The listing builds one solid part. Answer for the finished solid, in the listing's coordinates (mm). Face numbers are marked on the shaded views. Coordinates: 2 decimals unless noted, no trailing zeros. Loops run counter-clockwise (first coordinate to the right, second up) from the corner with the lowest first, then second, coordinate; pieces in that order, holes last. Notation, with made-up numbers: (52.5, -11.5) - (102.5, -11.5) arc R10 ccw to (102.5, -1.5) - close; hole circle Ø9 at (-6, -29). An arc over 180 degrees is marked (long way). One line per question, with ' | ' between items.
from build123d import *

# Parameters (mm, degrees)
SKETCH1_R           = 1.5
BOSS_EXTRUDE1_DEPTH = 7


with BuildPart() as part:
    # Sketch1 → Boss-Extrude1 (new body)
    with BuildSketch(Plane(origin=(0, 0, 0), x_dir=(1, 0, 0), z_dir=(0, 1, 0))):
        Polygon((2.886751346, 0), (1.443375673, 2.5), (-1.443375673, 2.5), (-2.886751346, 0), (-1.443375673, -2.5), (1.443375673, -2.5), align=None)
        Circle(SKETCH1_R, mode=Mode.SUBTRACT)
    extrude(amount=BOSS_EXTRUDE1_DEPTH)

    # Sketch5 → Cut-Revolve4 (revolve, cut)
    with BuildSketch(Plane.XY):
        with BuildLine():
            Line((-2.5, 0), (-2.886751346, 0))
            Line((-2.886751346, 0), (-2.886751346, 0.25))
            ThreePointArc((-2.886751346, 0.25), (-2.707962836, 0.102433581), (-2.5, 0))
        make_face()
        with BuildLine():
            Line((-2.886751346, 7), (-2.886751346, 6.75))
            ThreePointArc((-2.886751346, 6.75), (-2.707962836, 6.897566419), (-2.5, 7))
            Line((-2.5, 7), (-2.886751346, 7))
        make_face()
    revolve(axis=Axis((0, 7.426750378, 0), (0, -1, 0)), mode=Mode.SUBTRACT)


solid = part.part
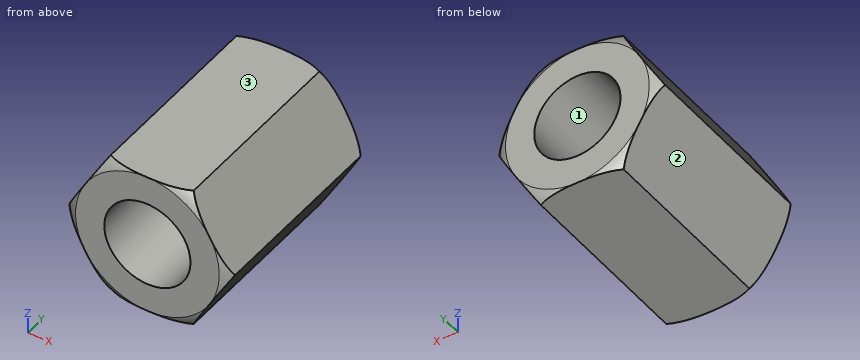
Item 1: Find the intervals of material crossed by line 1 (Z direction, x = 0, y = 4.25); line 2 (Z direction, x = 1.15, y = 2); line 3 (X direction, y = 3.25, z = 1.3), in increasing order. Write a range as [from, to].
Taken from the geometry:
line 1: z = [-2.5, -1.5], [1.5, 2.5] | line 2: z = [-2.5, -0.96], [0.96, 2.5] | line 3: x = [-2.14, -0.75], [0.75, 2.14]
Item 2: The mould has two halves that part along X. Classify the marked faces 1, 2 and 3: pulls with the +X half, pulls with the -X half, needs draft (parallel to the pull), parting line crosses it, or undercut.
Taken from the geometry:
face 1: undercut | face 2: pulls with the -X half | face 3: needs draft
Item 3: This flat-tipped pin is pushed along its axis until it touches: pin 1 Ø1.8 at (x, z) = (0, 0) entering from +Y. Where does it stop, or does it pass through?
Taken from the geometry:
pin 1: passes through
Item 4: Find section A-A, the plane y = 1. Write down the section's boundary in (x, z), plus the area to 3 significant figures.
Taken from the geometry:
outline: (-2.89, 0) - (-1.44, -2.5) - (1.44, -2.5) - (2.89, 0) - (1.44, 2.5) - (-1.44, 2.5) - close; hole circle Ø3 at (0, 0) | area: 14.6 mm2
